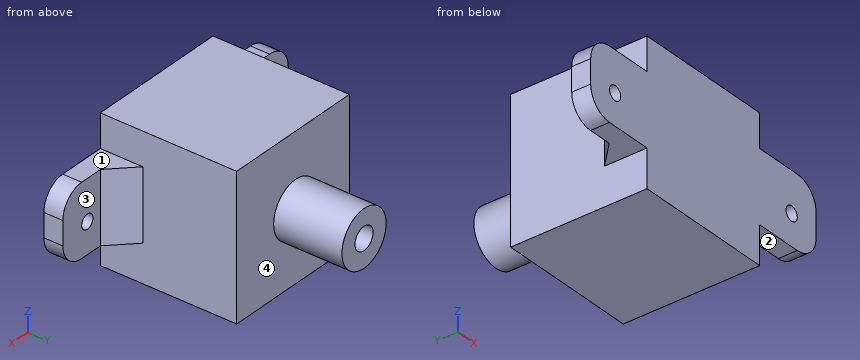
```python
from build123d import *

# Parameters (mm, degrees)
SKETCH_1_W               = 30
SKETCH_1_H               = 30
EXTRUDE_289_DEPTH        = 28.77
SKETCH_2_R               = 5.875
EXTRUDE_2_DEPTH          = 14.4
EXTRUDE_4_DEPTH          = 4
CUT_EXTRUDE_2_DEPTH      = 53.090646066
CUT_EXTRUDE_2_DEPTH_BACK = 53.090646066
SKETCH_6_R               = 1.5
CHAMFER_2_SIZE           = 5
CHAMFER_3_SIZE           = 5
SKETCH_4_R               = 2.4
CUT_EXTRUDE_3_DEPTH      = 8


with BuildPart() as part:
    # Эскиз1 → Extrude 289 (new body)
    with BuildSketch(Plane(origin=(0, 0, 0), x_dir=(1, 0, 0), z_dir=(0, 1, 0))):
        with Locations((0.713469456, -0.356734728)):
            Rectangle(SKETCH_1_W, SKETCH_1_H)
    extrude(amount=EXTRUDE_289_DEPTH)

    # Эскиз2 → Бобышка-Вытянуть2 (add)
    with BuildSketch(Plane(origin=(0, 28.77, 0), x_dir=(1, 0, 0), z_dir=(0, 1, 0))):
        with Locations(Location((0, 0, 0), (0, 0, 270))):
            Circle(SKETCH_2_R)
    extrude(amount=EXTRUDE_2_DEPTH)

    # Эскиз5 → Бобышка-Вытянуть4 (add)
    with BuildSketch(Plane.XZ):
        with BuildLine():
            Line((15.713469456, 8.356734728), (25.713469456, 8.356734728))
            ThreePointArc((25.713469456, 8.356734728), (29.249003362, 6.892268634), (30.713469456, 3.356734728))
            Line((30.713469456, 3.356734728), (30.713469456, -1.643265272))
            ThreePointArc((30.713469456, -1.643265272), (29.249003362, -5.178799178), (25.713469456, -6.643265272))
            Line((25.713469456, -6.643265272), (15.713469456, -6.643265272))
            Line((15.713469456, -6.643265272), (15.713469456, 8.356734728))
        make_face()
        with BuildLine():
            Line((-14.286530544, 8.356734728), (-24.286530544, 8.356734728))
            ThreePointArc((-24.286530544, 8.356734728), (-27.82206445, 6.892268634), (-29.286530544, 3.356734728))
            Line((-29.286530544, 3.356734728), (-29.286530544, -1.643265272))
            ThreePointArc((-29.286530544, -1.643265272), (-27.82206445, -5.178799178), (-24.286530544, -6.643265272))
            Line((-24.286530544, -6.643265272), (-14.286530544, -6.643265272))
            Line((-14.286530544, -6.643265272), (-14.286530544, 8.356734728))
        make_face()
    extrude(amount=-EXTRUDE_4_DEPTH)

    # Эскиз6 → Вырез-Вытянуть2 (cut, two sides: drawn at the far end of the back side and taken through both)
    with BuildSketch(Plane(origin=(0, 4, 0), x_dir=(1, 0, 0), z_dir=(0, 1, 0)).offset(-CUT_EXTRUDE_2_DEPTH_BACK)):
        with Locations(Location((24.213469456, 0.143265272, 0), (0, 0, 270))):
            Circle(SKETCH_6_R)
        with Locations(Location((-22.786530544, 0.143265272, 0), (0, 0, 270))):
            Circle(SKETCH_6_R)
    extrude(amount=CUT_EXTRUDE_2_DEPTH + CUT_EXTRUDE_2_DEPTH_BACK, mode=Mode.SUBTRACT)

    # Фаска2
    chamfer_2_edges = [part.edges().sort_by_distance(p)[0] for p in [
        (15.713469456, 4, 0.856734728),
    ]]
    chamfer(chamfer_2_edges, length=CHAMFER_2_SIZE)

    # Фаска3
    chamfer_3_edges = [part.edges().sort_by_distance(p)[0] for p in [
        (-14.286530544, 4, 0.856734728),
    ]]
    chamfer(chamfer_3_edges, length=CHAMFER_3_SIZE)

    # Эскиз4 → Вырез-Вытянуть3 (cut)
    with BuildSketch(Plane(origin=(0, 43.17, 0), x_dir=(1, 0, 0), z_dir=(0, 1, 0))):
        with Locations(Location((0, 0, 0), (0, 0, 270))):
            Circle(SKETCH_4_R)
    extrude(amount=-CUT_EXTRUDE_3_DEPTH, mode=Mode.SUBTRACT)


solid = part.part
```
Model file for the job. Use its own axes, mm. Face numbers are marked on the shaded views. A direction names the side the tool comes from. Coordinates: 2 decimals unless noted, no trailing zeros. Write each loop counter-clockwise with the first axis right and the second up, starting at its lowest first coordinate (ties: lowest second). Pieces come first, ordered by that corner, then holes. Notation, with made-up numbers: (-23.5, 7.25) - (-9.5, 7.25) arc R35 cw to (-9.5, 41.25) - close; hole circle Ø4 at (-16.75, 9.5). An arc over 180 degrees is marked (long way). One line per item, written item: value. Start each with the question number.
1. Slice it at D-D (z = -11.5). Write the cut outline in (x, y), plus the area to 3 significant figures.
2. Slice it at C-C (y = 38). Write the cut outline in (x, z) (3 decimals).
3. Tool access for the marked faces 1, 2, 3 and 4: list every direction of +Z, -Z, +X, -X, +Y, -Y with a clear straight run to the whole face (end or side of a thin tool).
4. Slice it at B-B (z = 0). Write the cut outline in (x, y) (3 decimals).
5. Flat gauge pins, fed straight in: pin 1 (1.5 mm diameter, centred on x = 19.5, y = 8.5, fed in from -Z); pin 2 (8 mm diameter, centred on y = 28.5, z = -1, fed in from +X); pin 3 (2.5 mm diameter, centred on x = -20, y = 3.5, fed in from -Z); pin 4 (1.4 mm diameter, centred on x = -0.5, z = 0, fed in from +Y). Where does each tip first touch, or does it go through?
6. Slice it at A-A (x = 0). Write the cut outline in (y, z) (3 decimals).
7. Probe line 1 (X direction, y = 2, z = 9.25); line 2 (Y direction, x = 15.5, z = 8); line 3 (X direction, y = 36, z = 0.75). List the from-to ranges inside material, lowest first. Write a range as from..to.
Answers below:
1. outline: (-14.29, 0) - (15.71, 0) - (15.71, 28.77) - (-14.29, 28.77) - close
1. area: 863 mm^2
2. outline: circle Ø11.75 at (0, 0); hole circle Ø4.8 at (0, 0)
3. face 1: +Z, +X, +Y, -Y
3. face 2: -Z, +X, +Y, -Y
3. face 3: +Z, -Z, +X, +Y
3. face 4: +Y
4. outline: (-29.287, 0) - (-24.28, 0) - (-24.28, 4) - (-29.287, 4) - close; (-21.293, 0) - (22.72, 0) - (22.72, 4) - (20.713, 4) - (15.713, 9) - (15.713, 28.77) - (5.875, 28.77) - (5.875, 43.17) - (2.4, 43.17) - (2.4, 35.17) - (-2.4, 35.17) - (-2.4, 43.17) - (-5.875, 43.17) - (-5.875, 28.77) - (-14.287, 28.77) - (-14.287, 9) - (-19.287, 4) - (-21.293, 4) - close; (25.707, 0) - (30.713, 0) - (30.713, 4) - (25.707, 4) - close
5. pin 1: passes through
5. pin 2: stops at x = 15.71
5. pin 3: stops at z = -6.64
5. pin 4: stops at y = 35.17
6. outline: (0, -14.643) - (28.77, -14.643) - (28.77, -5.875) - (43.17, -5.875) - (43.17, -2.4) - (35.17, -2.4) - (35.17, 2.4) - (43.17, 2.4) - (43.17, 5.875) - (28.77, 5.875) - (28.77, 15.357) - (0, 15.357) - close
7. line 1: x = -14.29..15.71
7. line 2: y = 0..28.77
7. line 3: x = -5.83..-2.28, 2.28..5.83
